from build123d import *

# Parameters (mm, degrees)
BOSS_EXTRUDE1_DEPTH        = 19.05
BOSS_EXTRUDE1_DEPTH_BACK   = 19.05
SKETCH3_W                  = 152.4
SKETCH3_H                  = 3.175
F_8_CLEARANCE_HOLE1_D      = 4.4958
F_6_0_204_DIAMETER_HOLE1_D = 5.1816


with BuildPart() as part:
    # Sketch3 → Boss-Extrude1 (new, two sides: drawn at the far end of the back side and taken through both)
    with BuildSketch(Plane.XY.offset(-BOSS_EXTRUDE1_DEPTH_BACK)):
        Rectangle(SKETCH3_W, SKETCH3_H)
    extrude(amount=BOSS_EXTRUDE1_DEPTH + BOSS_EXTRUDE1_DEPTH_BACK)

    # #8 Clearance Hole1 (through all)
    with Locations(Plane(origin=(0, 1.5875, 0), x_dir=(1, 0, 0), z_dir=(0, 1, 0))):
        with Locations((-69.85, 13.97), (-69.85, -13.97)):
            f_8_clearance_hole1 = Hole(F_8_CLEARANCE_HOLE1_D / 2)

    # Mirror1: #8 Clearance Hole1 across plane
    add(f_8_clearance_hole1.mirror(Plane(origin=(0, 0, 0), x_dir=(0, 0, 1), z_dir=(1, 0, 0))), mode=Mode.SUBTRACT)

    # #6 (0.204) Diameter Hole1 (through all)
    with Locations(Plane(origin=(0, 1.5875, 0), x_dir=(1, 0, 0), z_dir=(0, 1, 0))):
        with Locations((0, 7.62)):
            Hole(F_6_0_204_DIAMETER_HOLE1_D / 2)


solid = part.part
Work out the finished part from the listing and answer in its coordinate system (mm). Round coordinates to 2 decimals unless told otherwise and drop trailing zeros. Order: outer loops, then holes, each group sorted by start corner. A loop starts at its lowest first (then second) coordinate and runs counter-clockwise, first axis right, second up. Notation, with made-up numbers: M -4.5,61 L 43.5,61 A24 ccw 43.5,71 Z; hole C -2,51 d7. An arc over 180 degrees is marked long. Put each result on its own line as item: value. Start each with the question number.
Q1. Straight lines are drawn through the part: L1, parallel to Z at x = 69.85, y = -0.75; L2, parallel to Z at x = 0, y = 0.3; L3, parallel to X at y = 1.35, z = 16. For each, find the intervals that lie inside material, in ascending order. Write a range as [from, to].
Q2. For a pull along X with two mould halves and no side action, classify faces 1 (the flat face through (-1, 0, -19.05)), 2 (the flat face through (76.2, 0, 0)), 3 (the cylindrical face through (-71.994, -0.022, 13.295)) as pulls with the +X half, pulls with the -X half, needs draft (parallel to the pull), parting line crosses it, or undercut.
Q3. Section C-C, the plane z = -13.97 is taken. Write down the section's boundary in (x, y), and give its area (3 significant figures).
Q4. Section B-B, the plane x = 69.85 is taken. Write down the section's boundary in (y, z), and give its area (3 significant figures).
Q5. Section A-A, the plane x = 0 is taken. Write down the section's boundary in (y, z).
Q6. Flat-ended cylindrical pins translate along their axes: pin 1 (4 mm diameter, centred on x = 0, z = -7.62, fed in from +Y); pin 2 (7 mm diameter, centred on x = 69.85, z = 13.97, fed in from -Y). Find the tip coordinate at first contact, or state that the pin passes through.
Q7. Section D-D, the plane z = -7.62 is taken. Write down the section's boundary in (x, y).
Findings below:
1. L1: z = [-19.05, -16.22], [-11.72, 11.72], [16.22, 19.05]
1. L2: z = [-19.05, -10.21], [-5.03, 19.05]
1. L3: x = [-76.2, -70.82], [-68.88, 68.88], [70.82, 76.2]
2. face 1: needs draft
2. face 2: pulls with the +X half
2. face 3: undercut
3. outline: M -76.2,-1.59 L -72.1,-1.59 L -72.1,1.59 L -76.2,1.59 Z; M -67.6,-1.59 L 67.6,-1.59 L 67.6,1.59 L -67.6,1.59 Z; M 72.1,-1.59 L 76.2,-1.59 L 76.2,1.59 L 72.1,1.59 Z
3. area: 455 mm^2
4. outline: M -1.59,-19.05 L 1.59,-19.05 L 1.59,-16.22 L -1.59,-16.22 Z; M -1.59,-11.72 L 1.59,-11.72 L 1.59,11.72 L -1.59,11.72 Z; M -1.59,16.22 L 1.59,16.22 L 1.59,19.05 L -1.59,19.05 Z
4. area: 92.4 mm^2
5. outline: M -1.59,-19.05 L 1.59,-19.05 L 1.59,-10.21 L -1.59,-10.21 Z; M -1.59,-5.03 L 1.59,-5.03 L 1.59,19.05 L -1.59,19.05 Z
6. pin 1: passes through
6. pin 2: stops at y = -1.59
7. outline: M -76.2,-1.59 L -2.59,-1.59 L -2.59,1.59 L -76.2,1.59 Z; M 2.59,-1.59 L 76.2,-1.59 L 76.2,1.59 L 2.59,1.59 Z
